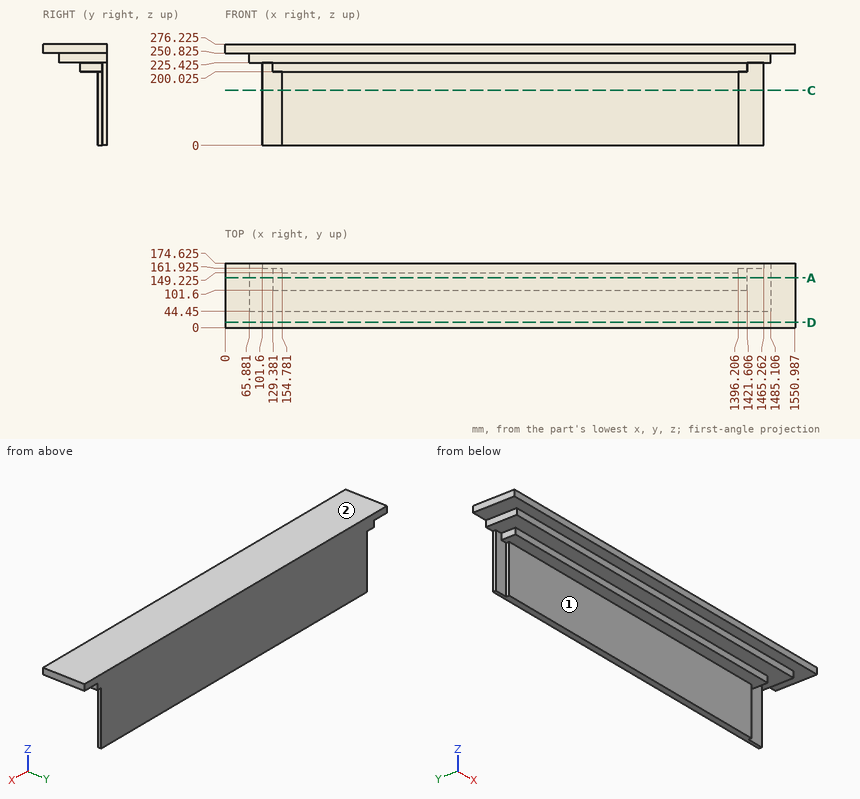
Design review of the part shown in the three views and the two pictorial views. Dimensions are in mm from the part's minimum x, y and z. A direction names the side the tool comes from. Round coordinates to 2 decimals unless told otherwise and drop trailing zeros. Write each loop counter-clockwise with the first axis right and the second up, starting at its lowest first coordinate (ties: lowest second). Pieces come first, ordered by that corner, then holes. Notation, with made-up numbers: M 0.5,84.5 L 59.5,84.5 A6 cw 59.5,94.5 Z; hole C 69.25,12 d5. An arc over 180 degrees is marked long. One line per item, written item: value. Start each with the question number.
1. Take a section at A-A on y = 135.5. State the section outline as (x, z) points (1 decimal), then the cut area to 3 significant figures.
2. For the marked faces 1 and 2, list the 3-axis set-ups (+Z, -Z, +X, -X, +Y, -Y) from which the entire face can be reached by the end or side of a thin tool; tool diameter is ignored.
3. Take a section at C-C on z = 150. State the section outline as (x, y) points (1 decimal), then the cut area to 3 significant figures.
4. To check wall thickness, follow probe 1 along Y at (x, z) = (509.5, 12) (1 decimal); probe 2 along Z at (x, y) = (257, 104) (1 decimal); probe 3 along X at (y, z) = (101, 240). State the ranges of each line that lie inside material, in increasing order. Write a range as from..to.
5. Clearance check with flat-ended pins moving along their axes: P1, Ø3, axis at x = 441, z = 65.5, coming from the -Y side (1 decimal); P2, Ø7.5, axis at y = 121, z = 212.5, coming from the +X side; P3, Ø7.5, axis at y = 98, z = 242, coming from the +X side. State where each tip first meets the part, or that it passes through.
6. Take a section at D-D on y = 14.5. State the section outline as (x, z) points (1 decimal), then the cut area to 3 significant figures.
Computed:
1. outline: M 0,250.8 L 65.9,250.8 L 65.9,225.4 L 129.4,225.4 L 129.4,200 L 1421.6,200 L 1421.6,225.4 L 1485.1,225.4 L 1485.1,250.8 L 1551,250.8 L 1551,276.2 L 0,276.2 Z
1. area: 108,000 mm²
2. face 1: -Z, +X, -X, -Y
2. face 2: +Z, +X, -X, +Y, -Y
3. outline: M 101.6,161.9 L 154.8,161.9 L 154.8,149.2 L 1396.2,149.2 L 1396.2,161.9 L 1465.3,161.9 L 1465.3,174.6 L 101.6,174.6 Z
3. area: 33,100 mm²
4. probe 1: y = 149.2..174.6
4. probe 2: z = 200..276.2
4. probe 3: x = 65.88..1485.11
5. P1: stops at y = 149.2
5. P2: stops at x = 1421.61
5. P3: stops at x = 1485.11
6. outline: M 0,250.8 L 1551,250.8 L 1551,276.2 L 0,276.2 Z
6. area: 39,400 mm²
